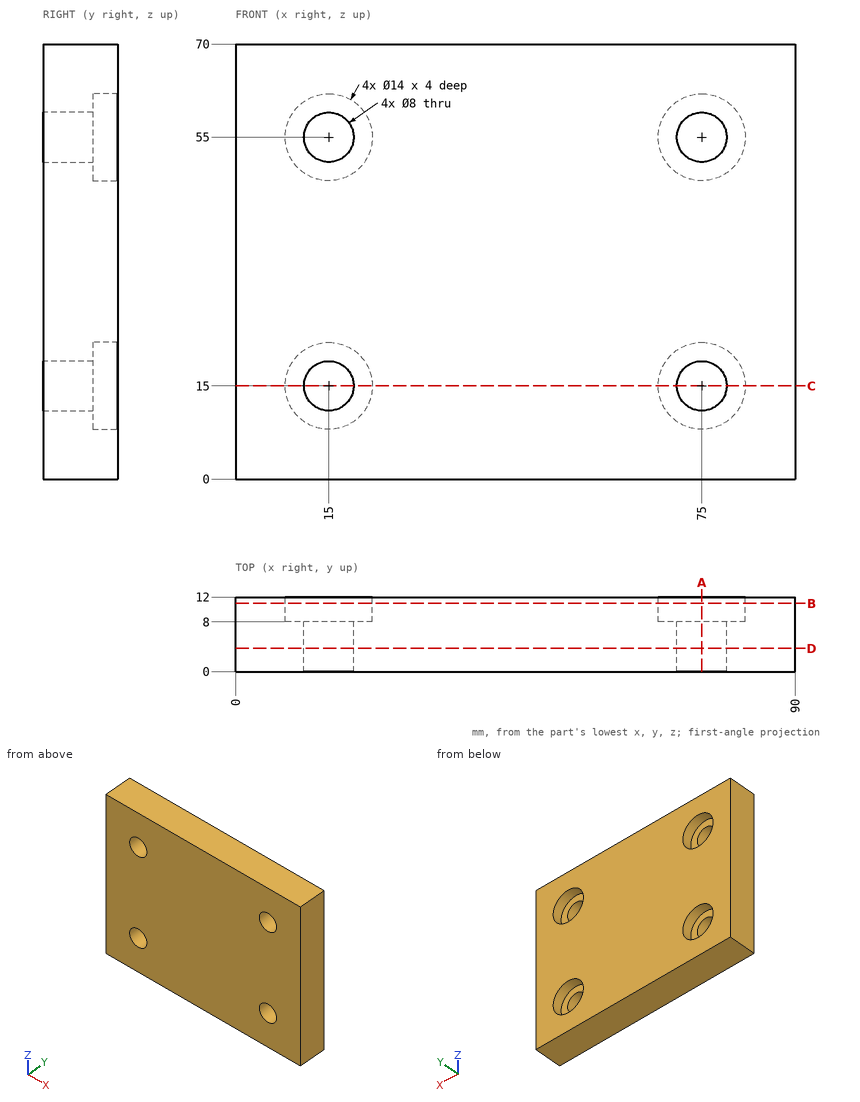
Here's the drawing with two shaded views (mm, measured from the low corner). I have some questions. Give positions to 0.01 mm unless a question says otherwise; leave off trailing zeros. Loops run counter-clockwise (first coordinate to the right, second up) from the corner with the lowest first, then second, coordinate; pieces in that order, holes last. Notation, with made-up numbers: (49.25, -5) -> (67.25, -5) arc R22 cw to (67.25, 29) -> close; hole circle Ø11 at (65.5, 38.5). An arc over 180 degrees is marked (long way). Answer as a JSON object with one key per item and string values. Group by question number.
Item 1: Will these pins go through, and if not, where does the flat tip stop? pin 1 (4 mm diameter, centred on x = 16.5, z = 12.5, fed in from +Y); pin 2 (6.5 mm diameter, centred on x = 15, z = 15, fed in from -Y).
Item 2: Imagine slicing it at D-D on y = 3.75. Write out the boundary of the cut face in (x, z).
Item 3: I need wall thicknesses on L1, parallel to X at y = 6.25, z = 15; L2, parallel to Z at x = 73, y = 7; L3, parallel to Z at x = 77.5, y = 7.75. Which ranges of each line are inside material? Lowest first, please.
Item 4: Imagine slicing it at A-A on x = 75. Write out the boundary of the cut face in (y, z).
Item 5: Imagine slicing it at B-B on y = 11. Write out the boundary of the cut face in (x, z).
Item 6: Imagine slicing it at C-C on z = 15. Write out the boundary of the cut face in (x, y), then the cut area to 3 significant figures.
Answer list:
{
 "1": {"pin 1": "stops at y = 8", "pin 2": "passes through"},
 "2": {"outline": "(0, 0) -> (90, 0) -> (90, 70) -> (0, 70) -> close; hole circle Ø8 at (15, 15); hole circle Ø8 at (15, 55); hole circle Ø8 at (75, 15); hole circle Ø8 at (75, 55)"},
 "3": {"L1": "x = 0 to 11, 19 to 71, 79 to 90", "L2": "z = 0 to 11.54, 18.46 to 51.54, 58.46 to 70", "L3": "z = 0 to 11.88, 18.12 to 51.88, 58.12 to 70"},
 "4": {"outline": "(0, 0) -> (12, 0) -> (12, 8) -> (8, 8) -> (8, 11) -> (0, 11) -> close; (0, 19) -> (8, 19) -> (8, 22) -> (12, 22) -> (12, 48) -> (8, 48) -> (8, 51) -> (0, 51) -> close; (0, 59) -> (8, 59) -> (8, 62) -> (12, 62) -> (12, 70) -> (0, 70) -> close"},
 "5": {"outline": "(0, 0) -> (90, 0) -> (90, 70) -> (0, 70) -> close; hole circle Ø14 at (15, 15); hole circle Ø14 at (15, 55); hole circle Ø14 at (75, 15); hole circle Ø14 at (75, 55)"},
 "6": {"outline": "(0, 0) -> (11, 0) -> (11, 8) -> (8, 8) -> (8, 12) -> (0, 12) -> close; (19, 0) -> (71, 0) -> (71, 8) -> (68, 8) -> (68, 12) -> (22, 12) -> (22, 8) -> (19, 8) -> close; (79, 0) -> (90, 0) -> (90, 12) -> (82, 12) -> (82, 8) -> (79, 8) -> close", "area": "840 mm2"}
}
